Build history of the part. All positions in model axes, mm. A direction names the side the tool comes from. Round coordinates to 2 decimals unless told otherwise and drop trailing zeros. Order: outer loops, then holes, each group sorted by start corner. A loop starts at its lowest first (then second) coordinate and runs counter-clockwise, first axis right, second up. Notation, with made-up numbers: (60, -3) - (85, -3) arc R25 cw to (85, 17) - close; hole circle Ø4 at (-15, -18). An arc over 180 degrees is marked (long way). One line per question, with ' | ' between items. Start each with the question number.
from build123d import *

# Parameters (mm, degrees)
F0_W     = 51.630139
F0_H     = 47.6119
F1_DEPTH = 25.4
F2_T     = -127
F3_T     = -2.54
F4_R     = 6.362452
F5_DEPTH = 25.4


with BuildPart() as f1:
    # F0 (on Front) → F1 (new body)
    with BuildSketch(Plane.XZ):
        with Locations((25.815069, 23.80595)):
            Rectangle(F0_W, F0_H)
    extrude(amount=F1_DEPTH)

    # F2
    f2_openings = [f1.faces().sort_by_distance(p)[0] for p in [
        (0, -12.7, 23.80595),
    ]]
    offset(amount=F2_T, openings=f2_openings)

    # F3
    f3_openings = [f1.faces().sort_by_distance(p)[0] for p in [
        (25.81507, -12.7, 0),
    ]]
    offset(amount=F3_T, openings=f3_openings)

    # F4 (on face) → F5 (join)
    with BuildSketch(Plane.XZ.offset(25.4)):
        with Locations((25.81507, 23.704037)):
            Circle(F4_R)
    extrude(amount=F5_DEPTH)


solid = f1.part
Item 1: Slice it at B-B (x = 8). Write the cut outline in (y, z), plus the area to 3 significant figures.
Item 2: Slice it at D-D (z = 33). Write the cut outline in (x, y).
Item 3: Wall check: line 1 along Y through (x, z) = (4.5, 6.5); line 2 along X through (y, z) = (-13.5, 22); line 3 along Z through (x, y) = (26.5, -17). Give the ranges that are in metal, low to high. Write a range as [from, to].
Item 4: Pin check, flat tips, straight feed: pin 1 (6 mm diameter, centred on x = 32.5, y = -13.5, fed in from -Z); pin 2 (1 mm diameter, centred on x = 26, y = -34.5, fed in from +Z); pin 3 (1 mm diameter, centred on x = 31.5, z = 16, fed in from -Y). Stop position of each tip, or through.
Item 5: Slice it at C-C (z = 25). Write the cut outline in (x, y), plus the area to 3 significant figures.
Item 6: Slice it at A-A (y = -10). Write the cut outline in (x, z).
Item 7: 3-axis set-ups, long thin cutter, end or side, ignore diameter. For faces 1 (the face through (26, -2, 0)), 2 (the face through (25, -2.54, 23)), 3 (the face through (31.884, -37.922, 25.615)): which of +Z, -Z, +X, -X, +Y, -Y reach the whole face in a straight line?
A:
1) outline: (-25.4, 0) - (-22.86, 0) - (-22.86, 45.07) - (-2.54, 45.07) - (-2.54, 0) - (0, 0) - (0, 47.61) - (-25.4, 47.61) - close | area: 293 mm^2
2) outline: (0, -25.4) - (51.63, -25.4) - (51.63, 0) - (0, 0) - close; hole (2.54, -22.86) - (49.09, -22.86) - (49.09, -2.54) - (2.54, -2.54) - close
3) line 1: [-25.4, -22.86], [-2.54, 0] | line 2: [0, 2.54], [49.09, 51.63] | line 3: [45.07, 47.61]
4) pin 1: z = 45.07 | pin 2: z = 30.07 | pin 3: y = -25.4
5) outline: (0, -25.4) - (19.59, -25.4) - (19.59, -50.8) - (32.04, -50.8) - (32.04, -25.4) - (51.63, -25.4) - (51.63, 0) - (0, 0) - close; hole (2.54, -22.86) - (49.09, -22.86) - (49.09, -2.54) - (2.54, -2.54) - close | area: 682 mm^2
6) outline: (0, 0) - (2.54, 0) - (2.54, 45.07) - (49.09, 45.07) - (49.09, 0) - (51.63, 0) - (51.63, 47.61) - (0, 47.61) - close
7) face 1: -Z, +X, -X, +Y, -Y | face 2: -Z | face 3: -Y
